from build123d import *

# Parameters (mm, degrees)
F0_W     = 27
F0_H     = 114
F1_DEPTH = 1
F0_W_2   = 18.1
F0_H_2   = 31.8
F2_DEPTH = 3
F3_R     = 3
F4_W     = 8
F4_H     = 108.75
F5_DEPTH = 2


with BuildPart() as f1:
    # F0 (on Top) → F1 (new body)
    with BuildSketch(Plane.XY):
        Rectangle(F0_W, F0_H)
        Polygon((9.05, 24.1), (10.275, 24.1), (10.275, -53.75), (-10.275, -53.75), (-10.275, 24.1), (-9.05, 24.1), (-9.05, 55.9), (9.05, 55.9), align=None, mode=Mode.SUBTRACT)
    extrude(amount=F1_DEPTH)

    # F0 (on Top) → F2 (join)
    with BuildSketch(Plane.XY):
        Polygon((10.275, -53.75), (10.275, 24.1), (9.05, 24.1), (-9.05, 24.1), (-10.275, 24.1), (-10.275, -53.75), align=None)
        with Locations((0, 40)):
            Rectangle(F0_W_2, F0_H_2)
    extrude(amount=F2_DEPTH)

    # F3
    f3_edges = [f1.edges().sort_by_distance(p)[0] for p in [
        (13.5, -57, 0.5),
        (-13.5, -57, 0.5),
        (13.5, 57, 0.5),
        (-13.5, 57, 0.5),
    ]]
    fillet(f3_edges, radius=F3_R)

    # F4 (on face) → F5 (cut)
    with BuildSketch(Plane.XY.offset(3)):
        with Locations((0, 0.625)):
            Rectangle(F4_W, F4_H)
    extrude(amount=-F5_DEPTH, mode=Mode.SUBTRACT)


solid = f1.part
The model under review builds one solid part; all positions refer to its coordinate system, in mm. A direction names the side the tool comes from. Give positions to 0.01 mm unless a question says otherwise; leave off trailing zeros. Write each loop counter-clockwise with the first axis right and the second up, starting at its lowest first coordinate (ties: lowest second). Pieces come first, ordered by that corner, then holes. Notation, with made-up numbers: M 67.5,26 L 100.5,26 A7 cw 100.5,33 Z; hole C 87,2.25 d1. An arc over 180 degrees is marked long. One line per question, with ' | ' between items. Start each with the question number.
Item 1: We need section C-C on z = 1.9. Write out the cut boundary in (x, y) (3 decimals).
Item 2: Wall thickness on line 1 (X direction, y = -38, z = 1.95) (3 decimals); line 2 (X direction, y = 31, z = 2.85); line 3 (Y direction, x = -9.75, z = 2.85): over which ranges is each line inside the solid? List them lowest first. Write a range as from..to.
Item 3: We need section A-A on x = -5. Write out the cut boundary in (y, z), plus the area to 3 significant figures.
Item 4: For pin 1 (0.6 mm diameter, centred on y = 45.5, z = 2.5, fed in from -X); pin 2 (1.6 mm diameter, centred on y = -6.5, z = 2, fed in from -X) (3 decimals); pin 3 (1.6 mm diameter, centred on x = -2.5, z = 2, fed in from +Y), all flat-tipped, find the tip position at first contact; note any pin that passes through.
Item 5: For faces 4 (the flat face through (-4, 0, 2)), 5 (the flat face through (-7, -53.75, 2)), 6 (the flat face through (0, 55.9, 2)), list the 3-axis set-ups (+Z, -Z, +X, -X, +Y, -Y) from which the entire face can be reached by the end or side of a thin tool; tool diameter is ignored.
Item 6: Draft analysis for pull direction X (two halves, no side actions). For faces 1 (the cylindrical face through (12.6, -56.14, 0.51)), 2 (the cylindrical face through (-12.64, -56.1, 0.51)), 3 (the flat face through (0, 55, 2)), state which applies: released by +X, released by -X, zero draft, split by the parting line, or undercut.
Item 7: We need section B-B on y = 39.5. Write out the cut boundary in (x, z).
Item 8: We need section D-D on x = 11.5. Write out the cut boundary in (y, z).
Results found:
1) outline: M -10.275,-53.75 L -4,-53.75 L -4,55 L 4,55 L 4,-53.75 L 10.275,-53.75 L 10.275,24.1 L 9.05,24.1 L 9.05,55.9 L -9.05,55.9 L -9.05,24.1 L -10.275,24.1 Z
2) line 1: x = -10.275..-4, 4..10.275 | line 2: x = -9.05..-4, 4..9.05 | line 3: y = -53.75..24.1
3) outline: M -57,0 L 57,0 L 57,1 L 55.9,1 L 55.9,3 L -53.75,3 L -53.75,1 L -57,1 Z | area: 333 mm2
4) pin 1: stops at x = -9.05 | pin 2: stops at x = -10.275 | pin 3: stops at y = 55.9
5) face 4: +Z, -Y | face 5: +Z, +X, -X, -Y | face 6: +Z, +X, -X, +Y
6) face 1: released by +X | face 2: released by -X | face 3: undercut
7) outline: M -13.5,0 L 13.5,0 L 13.5,1 L 9.05,1 L 9.05,3 L 4,3 L 4,1 L -4,1 L -4,3 L -9.05,3 L -9.05,1 L -13.5,1 Z
8) outline: M -56.83,0 L 56.83,0 L 56.83,1 L -56.83,1 Z
